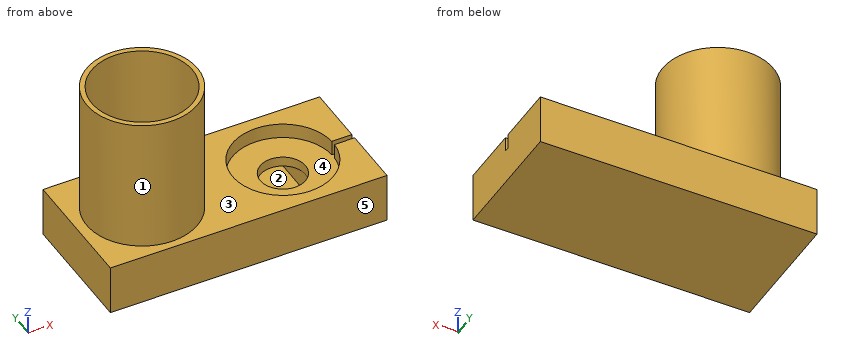
from build123d import *

# Parameters (mm, degrees)
F0_R          = 11
F0_R_2        = 10
F0_R_3        = 4.5
F1_DEPTH      = 3
F1_DEPTH_BACK = 7
F2_DEPTH      = 3
F3_DEPTH      = 6
F5_DEPTH      = 32.5
F6_DEPTH      = 30


with BuildPart() as f1:
    # F0 (on Top) → F1 (new body, two sides)
    with BuildSketch(Plane.XY) as f1_sk:
        with BuildLine():
            ThreePointArc((37.9874921777, -0.5), (18, 0), (37.9874921777, 0.5))
            Line((37.9874921777, 0.5), (42, 0.5))
            Line((42, 0.5), (42, 12.5))
            Line((42, 12.5), (-13, 12.5))
            Line((-13, 12.5), (-13, -12.5))
            Line((-13, -12.5), (42, -12.5))
            Line((42, -12.5), (42, -0.5))
            Line((42, -0.5), (37.9874921777, -0.5))
        make_face()
        Circle(F0_R, mode=Mode.SUBTRACT)
        Circle(F0_R)
        Circle(F0_R_2, mode=Mode.SUBTRACT)
        with BuildLine():
            ThreePointArc((37.9874921777, -0.5), (37.9968725554, -0.2500782106), (38, 0))
            ThreePointArc((38, 0), (37.9968725554, 0.2500782106), (37.9874921777, 0.5))
            ThreePointArc((37.9874921777, 0.5), (18, 0), (37.9874921777, -0.5))
        make_face()
        with Locations((28, 0)):
            Circle(F0_R_3, mode=Mode.SUBTRACT)
        Circle(F0_R_2)
        with Locations((28, 0)):
            Circle(F0_R_3)
        with BuildLine():
            ThreePointArc((37.9874921777, 0.5), (37.9968725554, 0.2500782106), (38, 0))
            Line((38, 0), (42, 0))
            Line((42, 0), (42, 0.5))
            Line((42, 0.5), (37.9874921777, 0.5))
        make_face()
        with BuildLine():
            Line((42, 0), (38, 0))
            ThreePointArc((38, 0), (37.9968725554, -0.2500782106), (37.9874921777, -0.5))
            Line((37.9874921777, -0.5), (42, -0.5))
            Line((42, -0.5), (42, 0))
        make_face()
    extrude(amount=F1_DEPTH)
    extrude(f1_sk.sketch, amount=-F1_DEPTH_BACK)

    # F0 (on Top) → F2 (cut)
    with BuildSketch(Plane.XY):
        Circle(F0_R_2)
        with BuildLine():
            ThreePointArc((37.9874921777, -0.5), (37.9968725554, -0.2500782106), (38, 0))
            ThreePointArc((38, 0), (37.9968725554, 0.2500782106), (37.9874921777, 0.5))
            ThreePointArc((37.9874921777, 0.5), (18, 0), (37.9874921777, -0.5))
        make_face()
        with Locations((28, 0)):
            Circle(F0_R_3, mode=Mode.SUBTRACT)
        with Locations((28, 0)):
            Circle(F0_R_3)
        with BuildLine():
            Line((42, 0), (38, 0))
            ThreePointArc((38, 0), (37.9968725554, -0.2500782106), (37.9874921777, -0.5))
            Line((37.9874921777, -0.5), (42, -0.5))
            Line((42, -0.5), (42, 0))
        make_face()
        with BuildLine():
            ThreePointArc((37.9874921777, 0.5), (37.9968725554, 0.2500782106), (38, 0))
            Line((38, 0), (42, 0))
            Line((42, 0), (42, 0.5))
            Line((42, 0.5), (37.9874921777, 0.5))
        make_face()
    extrude(amount=F2_DEPTH, mode=Mode.SUBTRACT)

    # F0 (on Top) → F3 (cut)
    with BuildSketch(Plane.XY):
        with Locations((28, 0)):
            Circle(F0_R_3)
        Circle(F0_R_2)
    extrude(amount=-F3_DEPTH, mode=Mode.SUBTRACT)

    # F4 (on Right) → F5 (cut)
    with BuildSketch(Plane.YZ):
        Polygon((10, -5), (10, -2), (-10, -2), (-10, -6), (10, -6), align=None)
    extrude(amount=F5_DEPTH, mode=Mode.SUBTRACT)

    # F0 (on Top) → F6 (join)
    with BuildSketch(Plane.XY):
        Circle(F0_R)
        Circle(F0_R_2, mode=Mode.SUBTRACT)
    extrude(amount=F6_DEPTH)


solid = f1.part
Geometry: final body of the model. Coordinates: model frame, mm. Face numbers are marked on the shaded views. A direction names the side the tool comes from. Round coordinates to 2 decimals unless told otherwise and drop trailing zeros. Loops run counter-clockwise (first coordinate to the right, second up) from the corner with the lowest first, then second, coordinate; pieces in that order, holes last.
Q1. Access query for the marked faces 4 and 5. Directions: +Z, -Z, +X, -X, +Y, -Y. A direction counts if a zero-diameter tool reaches every point of the face in a straight line with its end or side. Return the directions, or none.
Q2. Pin query (flat end, axial travel): P1, Ø10, axis at x = -3.5, z = 17, coming from the +Y side; P2, Ø3, axis at x = 2.5, y = 1.5, coming from the +Z side; P3, Ø4, axis at x = 30, y = 3, coming from the +Z side; P4, Ø12.5, axis at x = 14, y = -6, coming from the +Z side. Return the tip coordinate at first contact, or that it passes through.
Q3. Material intervals for L1, parallel to Z at x = 15, y = 1.75; L2, parallel to X at y = 0, z = 21; L3, parallel to Z at x = 24.5, y = 6.5, sorted ascending.
Q4. Section A-A on x = 15.5. Return loops of the section in (y, z).
Q5. Pull-direction query (Y, two-part tool) for the marked faces 1, 2 and 3; classes: released by +Y, released by -Y, zero draft, split by the parting line, or undercut.
Q6. Section B-B on y = 2.5. Return loops of the section in (x, z).
Q7. Section C-C on z = 6. Return loops of the section in (x, y), plus the area to 3 significant figures.
Q8. Section D-D on x = 28. Return loops of the section in (y, z), plus the area to 3 significant figures.
Evaluation:
1. face 4: +Z
1. face 5: +Z, -Z, +X, -X, -Y
2. P1: stops at y = 11
2. P2: stops at z = -6
2. P3: stops at z = 0
2. P4: stops at z = 30
3. L1: z = -7 to -6, -2 to 3
3. L2: x = -11 to -10, 10 to 11
3. L3: z = -7 to -6, -2 to 0
4. outline: (-12.5, -7) - (12.5, -7) - (12.5, 3) - (-12.5, 3) - close; hole (-10, -6) - (10, -6) - (10, -2) - (-10, -2) - close
5. face 1: split by the parting line
5. face 2: undercut
5. face 3: zero draft
6. outline: (-13, -7) - (42, -7) - (42, 3) - (37.68, 3) - (37.68, 0) - (31.74, 0) - (31.74, -2) - (32.5, -2) - (32.5, -6) - (-9.68, -6) - (-9.68, 30) - (-10.71, 30) - (-10.71, 3) - (-13, 3) - close; (9.68, -2) - (24.26, -2) - (24.26, 0) - (18.32, 0) - (18.32, 3) - (10.71, 3) - (10.71, 30) - (9.68, 30) - close
7. outline: circle Ø22 at (0, 0); hole circle Ø20 at (0, 0)
7. area: 66.0 mm2
8. outline: (-12.5, -7) - (12.5, -7) - (12.5, 3) - (10, 3) - (10, 0) - (4.5, 0) - (4.5, -2) - (10, -2) - (10, -6) - (-10, -6) - (-10, -2) - (-4.5, -2) - (-4.5, 0) - (-10, 0) - (-10, 3) - (-12.5, 3) - close
8. area: 92.0 mm2
